Part model, mm, in its own coordinate system. A direction names the side the tool comes from. Round coordinates to 2 decimals unless told otherwise and drop trailing zeros. Write each loop counter-clockwise with the first axis right and the second up, starting at its lowest first coordinate (ties: lowest second). Pieces come first, ordered by that corner, then holes.
```python
from build123d import *

# Parameters (mm, degrees)
SKETCH_1_W               = 90
SKETCH_1_H               = 50
SM_BASE_FLANGE_1_DEPTH   = 2
EXTRUDE_1_DEPTH          = 23
SKETCH_5_3_W             = 86
SKETCH_5_3_H             = 2
EXTRUDE_2_DEPTH          = 10
SKETCH_10_W              = 2
SKETCH_10_H              = 50
EXTRUDE_3_DEPTH          = 17.5
CUT_EXTRUDE_1_DEPTH      = 72.807033082
FILLET_1_R               = 1
SKETCH_12_R              = 3.1
CUT_EXTRUDE_2_DEPTH      = 72.807033082
SKETCH_13_R              = 3.1
CUT_EXTRUDE_3_DEPTH      = 72.807033082
MIRROR_5_COPY_1_SKETCH_R = 3.1
MIRROR_5_COPY_1_DEPTH    = 72.807033082
MIRROR_5_COPY_2_SKETCH_R = 3.1
MIRROR_5_COPY_2_DEPTH    = 72.807033082


# Sheet-metal steps are written as plain solids
with BuildPart() as part:
    # Sketch 1 → 基体-法兰1 (new body)
    with BuildSketch(Plane.XY):
        Rectangle(SKETCH_1_W, SKETCH_1_H)
    extrude(amount=-SM_BASE_FLANGE_1_DEPTH)

    # 草图5 → 凸台-拉伸1 (add)
    with BuildSketch(Plane(origin=(0, 0, -2), x_dir=(-1, 0, 0), z_dir=(0, 0, -1))):
        Polygon((-43, 25), (-45, 25), (-45, -25), (-43, -25), (-43, -23), (-43, 23), align=None)
        Polygon((45, 25), (43, 25), (43, 23), (43, -23), (43, -25), (45, -25), align=None)
    extrude(amount=EXTRUDE_1_DEPTH)

    # 草图5<3> → 凸台-拉伸2 (add)
    with BuildSketch(Plane(origin=(0, 0, -2), x_dir=(-1, 0, 0), z_dir=(0, 0, -1))):
        with Locations((0, 24)):
            Rectangle(SKETCH_5_3_W, SKETCH_5_3_H)
        with Locations((0, -24)):
            Rectangle(SKETCH_5_3_W, SKETCH_5_3_H)
    extrude(amount=EXTRUDE_2_DEPTH)

    # 草图10 → 凸台-拉伸3 (add)
    with BuildSketch(Plane.ZY.offset(45)):
        with Locations((-24, 0)):
            Rectangle(SKETCH_10_W, SKETCH_10_H)
    extrude_3 = extrude(amount=EXTRUDE_3_DEPTH)

    # 草图11 → 切除-拉伸1 (cut, through all)
    with BuildSketch(Plane(origin=(0, 0, -25), x_dir=(-1, 0, 0), z_dir=(0, 0, -1))):
        Polygon((57.5, 25), (62.5, 20), (62.5, 25), align=None)
        Polygon((57.5, -25), (62.5, -20), (62.5, -25), align=None)
    cut_extrude_1 = extrude(amount=-CUT_EXTRUDE_1_DEPTH, mode=Mode.SUBTRACT)

    # 镜向3: 凸台-拉伸3, 切除-拉伸1 across plane
    add(extrude_3.mirror(Plane(origin=(0, 0, 0), x_dir=(0, 0, 1), z_dir=(1, 0, 0))))
    add(cut_extrude_1.mirror(Plane(origin=(0, 0, 0), x_dir=(0, 0, 1), z_dir=(1, 0, 0))), mode=Mode.SUBTRACT)

    # 圆角1
    fillet_1_edges = [part.edges().sort_by_distance(p)[0] for p in [
        (-43, 0, -25),
        (-43, 0, -2),
        (43, 0, -2),
        (0, 23, -2),
        (0, -23, -2),
        (-45, 0, -23),
        (45, 0, -23),
        (0, 25, 0),
        (45, 0, 0),
        (0, -25, 0),
        (-45, 0, 0),
        (43, 0, -25),
    ]]
    fillet(fillet_1_edges, radius=FILLET_1_R)

    # 草图12 → 切除-拉伸2 (cut, through all)
    with BuildSketch(Plane(origin=(0, 0, -25), x_dir=(-1, 0, 0), z_dir=(0, 0, -1))):
        with Locations((-52.5, 15)):
            Circle(SKETCH_12_R)
    cut_extrude_2 = extrude(amount=-CUT_EXTRUDE_2_DEPTH, mode=Mode.SUBTRACT)

    # 草图13 → 切除-拉伸3 (cut, through all)
    with BuildSketch(Plane.XY):
        with Locations((23, 15)):
            Circle(SKETCH_13_R)
    cut_extrude_3 = extrude(amount=-CUT_EXTRUDE_3_DEPTH, mode=Mode.SUBTRACT)

    # 镜向4: 切除-拉伸2, 切除-拉伸3 across plane
    add(cut_extrude_2.mirror(Plane.ZX), mode=Mode.SUBTRACT)
    add(cut_extrude_3.mirror(Plane.ZX), mode=Mode.SUBTRACT)

    # 镜向5: 切除-拉伸2, 切除-拉伸3 across plane
    add(cut_extrude_2.mirror(Plane(origin=(0, 0, 0), x_dir=(0, 0, 1), z_dir=(1, 0, 0))), mode=Mode.SUBTRACT)
    add(cut_extrude_3.mirror(Plane(origin=(0, 0, 0), x_dir=(0, 0, 1), z_dir=(1, 0, 0))), mode=Mode.SUBTRACT)

    # 镜向5 copy 1 sketch → 镜向5 copy 1 (cut, through all)
    with BuildSketch(Plane(origin=(0, 0, -25), x_dir=(1, 0, 0), z_dir=(0, 0, -1))):
        with Locations((-52.5, 15)):
            Circle(MIRROR_5_COPY_1_SKETCH_R)
    extrude(amount=-MIRROR_5_COPY_1_DEPTH, mode=Mode.SUBTRACT)

    # 镜向5 copy 2 sketch → 镜向5 copy 2 (cut, through all)
    with BuildSketch(Plane(origin=(0, 0, 0), x_dir=(-1, 0, 0), z_dir=(0, 0, 1))):
        with Locations((23, 15)):
            Circle(MIRROR_5_COPY_2_SKETCH_R)
    extrude(amount=-MIRROR_5_COPY_2_DEPTH, mode=Mode.SUBTRACT)


solid = part.part
```
Q1. Cut at C-C on y = -5. Write the cut outline in (x, z).
Values follow:
outline: (-62.5, -25) - (-44, -25) arc R1 ccw to (-43, -24) - (-43, -3) arc R1 cw to (-42, -2) - (42, -2) arc R1 cw to (43, -3) - (43, -24) arc R1 ccw to (44, -25) - (62.5, -25) - (62.5, -23) - (46, -23) arc R1 cw to (45, -22) - (45, -1) arc R1 ccw to (44, 0) - (-44, 0) arc R1 ccw to (-45, -1) - (-45, -22) arc R1 cw to (-46, -23) - (-62.5, -23) - close
Q2. Cut at A-A on z = -20.5. Write the cut outline in (x, y).
Values follow:
outline: (-45, -25) - (-43, -25) - (-43, 25) - (-45, 25) - close; (43, -25) - (45, -25) - (45, 25) - (43, 25) - close
Q3. Wall check: L1, parallel to Y at x = 52.5, z = -24.2; L2, parallel to X at y = -15, z = -24.1; L3, parallel to X at y = -2, z = -4. Give the ranges that are in metal, low to high.
Values follow:
L1: y = -25 to -18.1, -11.9 to 11.9, 18.1 to 25
L2: x = -62.5 to -55.6, -49.4 to -43.01, 43.01 to 49.4, 55.6 to 62.5
L3: x = -45 to -43, 43 to 45
Q4. Which spindle directions (+Z, -Z, +X, -X, +Y, -Y) get a long thin tool onto all of the face, cutting with end or side? Do faces 5 (the flat face through (-45, 0, -11)), 6 (the cylindrical face through (-49.636, 13.813, -24.014)), 7 (the flat face through (54, 0, -23)), 8 (the flat face through (1, 23, -7)). Say none if no direction does.
Values follow:
face 5: +Z, -X, +Y, -Y
face 6: +Z, -Z
face 7: +Z, +X, +Y, -Y
face 8: -Z
Q5. Cut at B-B on x = -52.5. Write the cut outline in (y, z), plus the area to 3 significant figures.
Values follow:
outline: (-25, -25) - (-18.1, -25) - (-18.1, -23) - (-25, -23) - close; (-11.9, -25) - (11.9, -25) - (11.9, -23) - (-11.9, -23) - close; (18.1, -25) - (25, -25) - (25, -23) - (18.1, -23) - close
area: 75.2 mm2
Q6. Drop flat-ended pins along their axis: pin 1 (2 mm diameter, centred on x = 2.5, y = -23.5, fed in from -Z); pin 2 (1.5 mm diameter, centred on y = 11, z = -12.5, fed in from -X); pin 3 (22 mm diameter, centred on x = 18.5, y = -3, fed in from -Z). Give the stop position or say it passes through.
Values follow:
pin 1: stops at z = -12
pin 2: stops at x = -45
pin 3: stops at z = -2
Q7. Cut at D-D on x = 14. Write the cut outline in (y, z), plus the area to 3 significant figures.
Values follow:
outline: (-25, -12) - (-23, -12) - (-23, -3) arc R1 cw to (-22, -2) - (22, -2) arc R1 cw to (23, -3) - (23, -12) - (25, -12) - (25, -1) arc R1 ccw to (24, 0) - (-24, 0) arc R1 ccw to (-25, -1) - close
area: 140 mm2
Q8. Mould opens along Y. For faces 1 (the flat face through (60, -22.5, -24)), 2 (the cylindrical face through (-49.636, -13.813, -24.014)), 3 (the flat face through (53, 0, -25)), 4 (the cylindrical face through (-20.54, 13.114, -0.986)) say: +Y half, -Y half, draft (parallel to the pull), parting line (faces both ways), or undercut.
Values follow:
face 1: -Y half
face 2: undercut
face 3: draft
face 4: undercut
